Here's how the part is built. I have some questions about the finished solid (model axes, mm). Coordinates: 2 decimals unless noted, no trailing zeros. Write each loop counter-clockwise with the first axis right and the second up, starting at its lowest first coordinate (ties: lowest second). Pieces come first, ordered by that corner, then holes. Notation, with made-up numbers: (48, -37.5) -> (72, -37.5) arc R24 cw to (72, -5.5) -> close; hole circle Ø11 at (72.5, 49). An arc over 180 degrees is marked (long way). Put each result on its own line as item: value. Start each with the question number.
Item 1: I want a section at A-A, the plane x = -70. List the corners of the cut face in (y, z) for me.
Item 2: I want a section at B-B, the plane z = 2.9. List the corners of the cut face in (x, y) for me.
Item 3: I need wall thicknesses on line 1 (Y direction, x = -9.5, z = 2.5); line 2 (X direction, y = -40, z = 0.75); line 3 (Y direction, x = 27, z = 4). Which ranges of each line are inside material? Lowest first, please. Write a range as [from, to].
Item 4: If we mould it in two halves opening along X, with no side actions, what happens to faces 1 (the face through (33.523, -47.482, 2.465)), 2 (the face through (-80.618, 35.659, 2.535)), 3 (the face through (-24, -50.334, 2)), 4 (the face through (-66.847, -37.508, 2.535))? For each: released by +X, released by -X, zero draft, split by the parting line, or undercut.
from build123d import *

# Parameters (mm, degrees)
SKETCH_1_W          = 150
SKETCH_1_H          = 89
EXTRUDE_1_DEPTH     = 5
SKETCH_3_W          = 30
SKETCH_3_H          = 89
CUT_EXTRUDE_1_DEPTH = 5
SKETCH_4_R          = 2.75
CUT_EXTRUDE_2_DEPTH = 5
FILLET_2_R          = 10
SKETCH_5_R          = 1.5
CUT_EXTRUDE_7_DEPTH = 10


with BuildPart() as part:
    # 草图1 → 凸台-拉伸1 (new body)
    with BuildSketch(Plane.XY):
        with Locations((-8.469721768, -5.833878887)):
            Rectangle(SKETCH_1_W, SKETCH_1_H)
    extrude(amount=EXTRUDE_1_DEPTH)

    # 草图3 → 切除-拉伸1 (cut)
    with BuildSketch(Plane.XY.offset(5)):
        with Locations((51.530278232, -5.833878887)):
            Rectangle(SKETCH_3_W, SKETCH_3_H)
    extrude(amount=-CUT_EXTRUDE_1_DEPTH, mode=Mode.SUBTRACT)

    # 草图4 → 切除-拉伸2 (cut)
    with BuildSketch(Plane.XY.offset(5)):
        with Locations((-69.469721768, 26.666121113)):
            Circle(SKETCH_4_R)
        with Locations((-69.469721768, -38.333878887)):
            Circle(SKETCH_4_R)
        with Locations((22.530278232, 26.666121113)):
            Circle(SKETCH_4_R)
        with Locations((22.530278232, -38.333878887)):
            Circle(SKETCH_4_R)
    extrude(amount=-CUT_EXTRUDE_2_DEPTH, mode=Mode.SUBTRACT)

    # 圆角2
    fillet_2_edges = [part.edges().sort_by_distance(p)[0] for p in [
        (36.530278232, 38.666121113, 2.5),
        (36.530278232, -50.333878887, 2.5),
        (-83.469721768, 38.666121113, 2.5),
        (-83.469721768, -50.333878887, 2.5),
    ]]
    fillet(fillet_2_edges, radius=FILLET_2_R)

    # 草图5 → 切除-拉伸7 (cut)
    with BuildSketch(Plane(origin=(0, 0, 0), x_dir=(-1, 0, 0), z_dir=(0, 0, -1))):
        with Locations((9.519721768, -5.833878887)):
            Circle(SKETCH_5_R)
        with Locations((37.419721768, -5.833878887)):
            Circle(SKETCH_5_R)
    extrude(amount=-CUT_EXTRUDE_7_DEPTH, mode=Mode.SUBTRACT)


solid = part.part
Calculated:
1. outline: (-50.33, 0) -> (-41.03, 0) -> (-41.03, 5) -> (-50.33, 5) -> close; (-35.64, 0) -> (23.97, 0) -> (23.97, 5) -> (-35.64, 5) -> close; (29.36, 0) -> (38.67, 0) -> (38.67, 5) -> (29.36, 5) -> close
2. outline: (-83.47, -40.33) arc R10 ccw to (-73.47, -50.33) -> (26.53, -50.33) arc R10 ccw to (36.53, -40.33) -> (36.53, 28.67) arc R10 ccw to (26.53, 38.67) -> (-73.47, 38.67) arc R10 ccw to (-83.47, 28.67) -> close; hole circle Ø5.5 at (-69.47, -38.33); hole circle Ø5.5 at (-69.47, 26.67); hole circle Ø3 at (-37.42, -5.83); hole circle Ø3 at (-9.52, -5.83); hole circle Ø5.5 at (22.53, -38.33); hole circle Ø5.5 at (22.53, 26.67)
3. line 1: y = [-50.33, -7.33], [-4.33, 38.67]
3. line 2: x = [-83.47, -71.66], [-67.28, 20.34], [24.72, 36.53]
3. line 3: y = [-50.32, 38.66]
4. face 1: released by +X
4. face 2: released by -X
4. face 3: zero draft
4. face 4: undercut
